from build123d import *

# Parameters (mm, degrees)
PAD_DEPTH           = 20
POCKET_DEPTH        = 18.5
POCKET001_DEPTH     = 5
LINEARPATTERN_COUNT = 10
LINEARPATTERN_PITCH = 4.444444
PAD001_DEPTH        = 7.5
SKETCH004_R         = 1.69
POCKET002_DEPTH     = 6
SKETCH005_W         = 20
SKETCH005_H         = 4.8
POCKET003_DEPTH     = 0.6
SKETCH006_R         = 0.5
SKETCH006_W         = 10.6
SKETCH006_H         = 6
POCKET004_DEPTH     = 5


with BuildPart() as part:
    # Sketch → Pad (new body)
    with BuildSketch(Plane.XY):
        with BuildLine():
            Line((-15.5, 32), (15.5, 32))
            ThreePointArc((20.5, 27), (19.035534, 30.535534), (15.5, 32))
            Line((20.5, 27), (20.5, -27))
            ThreePointArc((15.5, -32), (19.035534, -30.535534), (20.5, -27))
            Line((15.5, -32), (-15.5, -32))
            ThreePointArc((-20.5, -27), (-19.035534, -30.535534), (-15.5, -32))
            Line((-20.5, -27), (-20.5, 27))
            ThreePointArc((-15.5, 32), (-19.035534, 30.535534), (-20.5, 27))
        make_face()
    extrude(amount=PAD_DEPTH)

    # Sketch001 (on Face10 of Pad) → Pocket (cut)
    with BuildSketch(Plane.XY.offset(20)):
        with BuildLine():
            Line((-15.5, 30), (15.5, 30))
            ThreePointArc((18.5, 27), (17.62132, 29.12132), (15.5, 30))
            Line((18.5, 27), (18.5, -27))
            ThreePointArc((15.5, -30), (17.62132, -29.12132), (18.5, -27))
            Line((15.5, -30), (-15.5, -30))
            ThreePointArc((-18.5, -27), (-17.62132, -29.12132), (-15.5, -30))
            Line((-18.5, -27), (-18.5, 27))
            ThreePointArc((-15.5, 30), (-17.62132, 29.12132), (-18.5, 27))
        make_face()
    extrude(amount=-POCKET_DEPTH, mode=Mode.SUBTRACT)

    # Sketch002 (on Face4 of Pocket) → Pocket001 (cut)
    with BuildSketch(Plane(origin=(0, 0, 0), x_dir=(1, 0, 0), z_dir=(0, 0, -1))):
        with BuildLine():
            ThreePointArc((-15, 21), (-16, 20), (-15, 19))
            Line((-15, 19), (15, 19))
            ThreePointArc((15, 19), (16, 20), (15, 21))
            Line((15, 21), (-15, 21))
        make_face()
    pocket001 = extrude(amount=-POCKET001_DEPTH, mode=Mode.SUBTRACT)

    # LinearPattern: Pocket001 ×10
    with Locations(*[(0, i * LINEARPATTERN_PITCH, 0) for i in range(1, LINEARPATTERN_COUNT)]):
        add(pocket001, mode=Mode.SUBTRACT)

    # Sketch003 (on Face59 of LinearPattern) → Pad001 (join)
    with BuildSketch(Plane.XY.offset(1.5)):
        with BuildLine():
            Line((-15.5, 30), (-11.5, 30))
            Line((-11.5, 30), (-11.5, 26))
            ThreePointArc((-14.5, 23), (-12.37868, 23.87868), (-11.5, 26))
            Line((-14.5, 23), (-18.5, 23))
            Line((-18.5, 23), (-18.5, 27))
            ThreePointArc((-15.5, 30), (-17.62132, 29.12132), (-18.5, 27))
        make_face()
        with BuildLine():
            Line((11.5, 30), (15.5, 30))
            ThreePointArc((18.5, 27), (17.62132, 29.12132), (15.5, 30))
            Line((18.5, 27), (18.5, 23))
            Line((18.5, 23), (14.5, 23))
            ThreePointArc((11.5, 26), (12.37868, 23.87868), (14.5, 23))
            Line((11.5, 26), (11.5, 30))
        make_face()
        with BuildLine():
            Line((-18.5, -23), (-14.5, -23))
            ThreePointArc((-11.5, -26), (-12.37868, -23.87868), (-14.5, -23))
            Line((-11.5, -26), (-11.5, -30))
            Line((-11.5, -30), (-15.5, -30))
            ThreePointArc((-18.5, -27), (-17.62132, -29.12132), (-15.5, -30))
            Line((-18.5, -27), (-18.5, -23))
        make_face()
        with BuildLine():
            Line((14.5, -23), (18.5, -23))
            Line((18.5, -23), (18.5, -27))
            ThreePointArc((15.5, -30), (17.62132, -29.12132), (18.5, -27))
            Line((15.5, -30), (11.5, -30))
            Line((11.5, -30), (11.5, -26))
            ThreePointArc((14.5, -23), (12.37868, -23.87868), (11.5, -26))
        make_face()
    extrude(amount=PAD001_DEPTH)

    # Sketch004 (on Face69 of Pad001) → Pocket002 (cut)
    with BuildSketch(Plane.XY.offset(9)):
        with Locations((15, 26.5)):
            Circle(SKETCH004_R)
        with Locations((-15, 26.5)):
            Circle(SKETCH004_R)
        with Locations((-15, -26.5)):
            Circle(SKETCH004_R)
        with Locations((15, -26.5)):
            Circle(SKETCH004_R)
    extrude(amount=-POCKET002_DEPTH, mode=Mode.SUBTRACT)

    # Sketch005 (on Face6 of Pocket002) → Pocket003 (cut)
    with BuildSketch(Plane.XZ.offset(32)):
        with Locations((0, 14.4)):
            Rectangle(SKETCH005_W, SKETCH005_H)
    extrude(amount=-POCKET003_DEPTH, mode=Mode.SUBTRACT)

    # Sketch006 (on Face6 of Pocket003) → Pocket004 (cut)
    with BuildSketch(Plane.XZ.offset(32)):
        with Locations((7.65, 14.4)):
            Circle(SKETCH006_R)
        with Locations((-7.65, 14.4)):
            Circle(SKETCH006_R)
        with Locations((0, 14.4)):
            Rectangle(SKETCH006_W, SKETCH006_H)
    extrude(amount=-POCKET004_DEPTH, mode=Mode.SUBTRACT)


solid = part.part
Part model, mm, in its own coordinate system. A direction names the side the tool comes from. Coordinates: 2 decimals unless noted, no trailing zeros. Write each loop counter-clockwise with the first axis right and the second up, starting at its lowest first coordinate (ties: lowest second). Pieces come first, ordered by that corner, then holes. Notation, with made-up numbers: M 23.5,-1.75 L 77.5,-1.75 A13 cw 77.5,16.25 Z; hole C 59.25,75.5 d7. An arc over 180 degrees is marked long. Return JSON: item names as keys, results as strings.
1. Saw through at C-C, the plane x = -9. Count the separate pieces of the cut face and the enclosed holes in it, then the cut area to 3 significant figures.
Determined:
{"separate pieces": "11", "enclosed holes": "0", "area": "137 mm²"}
2. Flat gauge pins, fed straight in: pin 1 Ø1 at (x, y) = (13.5, -9.5) entering from +Z; pin 2 Ø1.4 at (x, z) = (7.5, 13.5) entering from -Y; pin 3 Ø1 at (x, y) = (-14.5, 26) entering from +Z. Where does each tip first touch, or does it go through?
Determined:
{"pin 1": "z = 1.5", "pin 2": "y = -31.4", "pin 3": "z = 3"}
3. 3-axis set-ups, long thin cutter, end or side, ignore diameter. For faces 4 (the face through (0, 7.667, 1)), 5 (the face through (0, -32, 10)), 6 (the face through (-16.25, 27.64, 6.04)): which of +Z, -Z, +X, -X, +Y, -Y reach the whole face in a straight line?
Determined:
{"face 4": "+Z, -Z", "face 5": "+Z, -Z, +X, -X, -Y", "face 6": "+Z"}
4. Saw through at D-D, the plane z = 13. Write the cut outline in (x, y), then the cut area to 3 significant figures.
Determined:
{"outline": "M -20.5,-27 A5 ccw -15.5,-32 L -10,-32 L -10,-31.4 L -5.3,-31.4 L -5.3,-30 L -15.5,-30 A3 cw -18.5,-27 L -18.5,27 A3 cw -15.5,30 L 15.5,30 A3 cw 18.5,27 L 18.5,-27 A3 cw 15.5,-30 L 5.3,-30 L 5.3,-31.4 L 10,-31.4 L 10,-32 L 15.5,-32 A5 ccw 20.5,-27 L 20.5,27 A5 ccw 15.5,32 L -15.5,32 A5 ccw -20.5,27 Z", "area": "363 mm²"}
5. Saw through at B-B, the plane z = 18.75. Write the cut outline in (x, y), then the cut area to 3 significant figures.
Determined:
{"outline": "M -20.5,-27 A5 ccw -15.5,-32 L 15.5,-32 A5 ccw 20.5,-27 L 20.5,27 A5 ccw 15.5,32 L -15.5,32 A5 ccw -20.5,27 Z; hole M -18.5,-27 A3 ccw -15.5,-30 L 15.5,-30 A3 ccw 18.5,-27 L 18.5,27 A3 ccw 15.5,30 L -15.5,30 A3 ccw -18.5,27 Z", "area": "390 mm²"}
6. Saw through at A-A, the plane y = -20. Write the cut outline in (x, z), then the cut area to 3 significant figures.
Determined:
{"outline": "M -20.5,0 L -16,0 L -16,1.5 L -18.5,1.5 L -18.5,20 L -20.5,20 Z; M 16,0 L 20.5,0 L 20.5,20 L 18.5,20 L 18.5,1.5 L 16,1.5 Z", "area": "87.5 mm²"}
7. Probe L1, parallel to X at y = 5.5, z = 2; L2, parallel to X at y = -25, z = 3.5; L3, parallel to Z at x = 7.65, y = -31.1. List the from-to ranges inside material, lowest first.
Determined:
{"L1": "-20.5 to -18.5, 18.5 to 20.5", "L2": "-20.5 to -15.78, -14.22 to -11.67, 11.67 to 14.22, 15.78 to 20.5", "L3": "0 to 13.9, 14.9 to 20"}
8. Pull direction Z, two halves, no side cores. Call faces 1 (the face through (-12.36, -23.9, 5.2)), 2 (the face through (15, 27, 3)), 3 (the face through (0, -31, 17.4)): pulls with the +Z half, pulls with the -Z half, needs draft (parallel to the pull), parting line crosses it, or undercut.
Determined:
{"face 1": "needs draft", "face 2": "pulls with the +Z half", "face 3": "undercut"}
